Answer from the drawing. Dimensions are ordinates in mm from the lowest x, y and z of the part. Give positions to 0.01 mm unless a question says otherwise; leave off trailing zeros. Write each loop counter-clockwise with the first axis right and the second up, starting at its lowest first coordinate (ties: lowest second). Pieces come first, ordered by that corner, then holes. Notation, with made-up numbers: (63.5, 11) - (91.5, 11) arc R11 ccw to (91.5, 24) - close; hole circle Ø1 at (54.5, -27.75). An arc over 180 degrees is marked (long way). Answer as a JSON object with one key per item and string values. Group by question number.
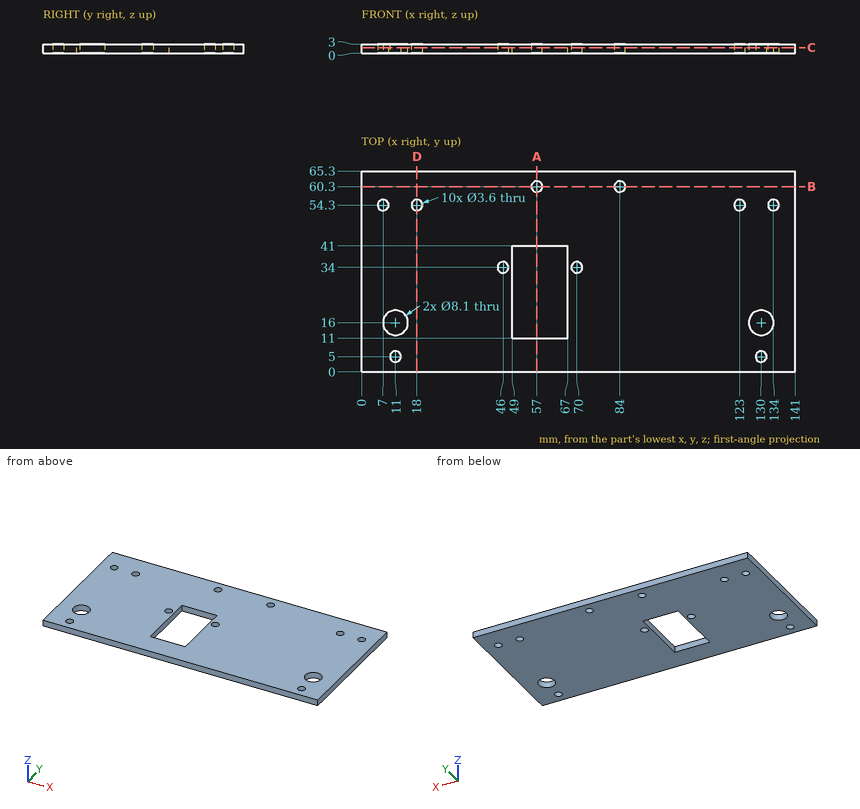
1) Find section B-B, the plane y = 60.3. Write down the section's boundary in (x, z).
2) A flat-ended cylindrical pin translates along its axis: pin 1 Ø3 at (x, y) = (7, 54.3) entering from +Z. Find the tip coordinate at first contact, or state that the pin passes through.
3) Find section D-D, the plane x = 18. Write down the section's boundary in (y, z), and give its area (3 significant figures).
4) Find the intervals of material crossed by line 1 (Y direction, x = 57, z = 1.45); line 2 (X direction, y = 27, z = 0.75); line 3 (Y direction, x = 11, z = 1.4), in increasing order. Write a range as [from, to].
5) Find section A-A, the plane x = 57. Write down the section's boundary in (y, z).
6) Find section C-C, the plane z = 1.8. Give the number of separate pieces and of enclosed holes in the cut face, and give its area (3 significant figures).
Values follow:
{
 "1": {"outline": "(0, 0) - (55.2, 0) - (55.2, 3) - (0, 3) - close; (58.8, 0) - (82.2, 0) - (82.2, 3) - (58.8, 3) - close; (85.8, 0) - (141, 0) - (141, 3) - (85.8, 3) - close"},
 "2": {"pin 1": "passes through"},
 "3": {"outline": "(0, 0) - (52.5, 0) - (52.5, 3) - (0, 3) - close; (56.1, 0) - (65.3, 0) - (65.3, 3) - (56.1, 3) - close", "area": "185 mm2"},
 "4": {"line 1": "y = [0, 11], [41, 58.5], [62.1, 65.3]", "line 2": "x = [0, 49], [67, 141]", "line 3": "y = [0, 3.2], [6.8, 11.95], [20.05, 65.3]"},
 "5": {"outline": "(0, 0) - (11, 0) - (11, 3) - (0, 3) - close; (41, 0) - (58.5, 0) - (58.5, 3) - (41, 3) - close; (62.1, 0) - (65.3, 0) - (65.3, 3) - (62.1, 3) - close"},
 "6": {"separate pieces": "1", "enclosed holes": "13", "area": "8,460 mm2"}
}
